Verification items for this drawing (mm, ordinates from the low corner). A direction names the side the tool comes from. Round coordinates to 2 decimals unless told otherwise and drop trailing zeros. Write each loop counter-clockwise with the first axis right and the second up, starting at its lowest first coordinate (ties: lowest second). Pieces come first, ordered by that corner, then holes. Notation, with made-up numbers: (-11.5, 26) -> (44.5, 26) arc R8 cw to (44.5, 31) -> close; hole circle Ø2 at (-6, 30.25). An arc over 180 degrees is marked (long way). One line per item, written item: value.
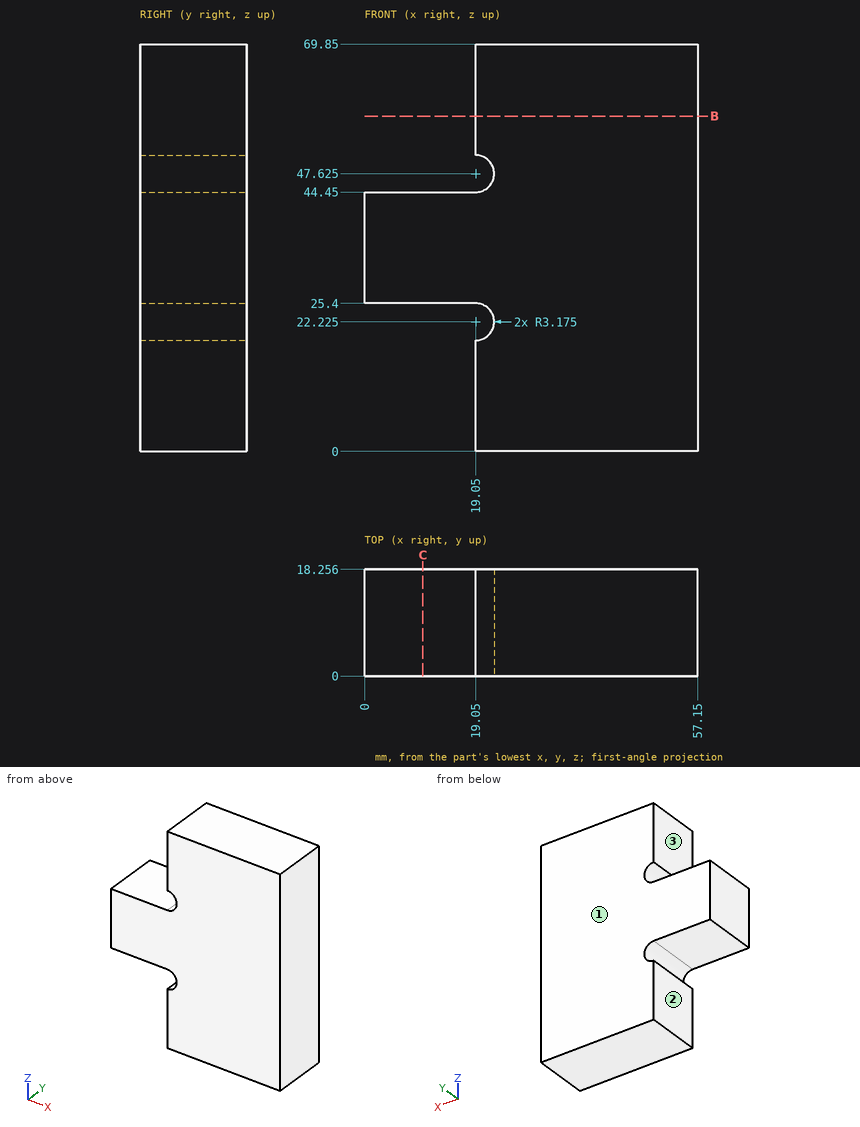
Item 1: Material ranges on line 1 along X through (y, z) = (16.5, 52); line 2 along Z through (x, y) = (4, 1); line 3 along X through (y, z) = (2.5, 46.5), recorded low to high.
Result set:
line 1: 19.05 to 57.15
line 2: 25.4 to 44.45
line 3: 22.02 to 57.15
Item 2: Sectioned sample at B-B (z = 57.5). Enter the section's corners in (x, y).
Result set:
outline: (19.05, 0) -> (57.15, 0) -> (57.15, 18.26) -> (19.05, 18.26) -> close
Item 3: Tool access check on the marked faces 1, 2 and 3. Record the directions out of +Z, -Z, +X, -X, +Y, -Y that give a thin tool (end or side, any length) a straight path to the whole face; none if there is none.
Result set:
face 1: +Z, -Z, +X, -X, +Y
face 2: -Z, -X, +Y, -Y
face 3: +Z, -X, +Y, -Y
Item 4: Depth check by flat-ended pin: pin 1 (3 mm diameter, centred on y = 2.5, z = 62, fed in from -X); pin 2 (9 mm diameter, centred on x = 12.5, y = 12.5, fed in from -Z); pin 3 (5.5 mm diameter, centred on x = 9.5, y = 8, fed in from +Z). Enter the tip coordinate at first touch or a pass-through.
Result set:
pin 1: x = 19.05
pin 2: z = 25.4
pin 3: z = 44.45
Item 5: Sectioned sample at C-C (x = 10). Enter the section's corners in (y, z).
Result set:
outline: (0, 25.4) -> (18.26, 25.4) -> (18.26, 44.45) -> (0, 44.45) -> close
